Work out the finished part from the listing and answer in its coordinate system (mm). Face numbers are marked on the shaded views. Coordinates: 2 decimals unless noted, no trailing zeros. Write each loop counter-clockwise with the first axis right and the second up, starting at its lowest first coordinate (ties: lowest second). Pieces come first, ordered by that corner, then holes. Notation, with made-up numbers: (22, 47.5) - (75, 47.5) arc R32 ccw to (75, 74.5) - close; hole circle Ø2 at (41, 22). An arc over 180 degrees is marked (long way). Answer as a JSON object with one key per item and string values. Group by question number.
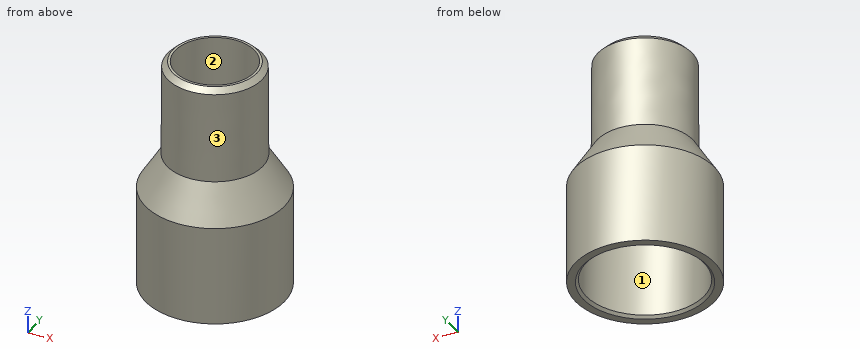
from build123d import *

# Parameters (mm, degrees)
F2_SIZE = 2
F3_SIZE = 1


with BuildPart() as f1:
    # F0 (on Front) → F1 (revolve)
    with BuildSketch(Plane.XZ):
        Polygon((22.5, 38), (22.5, 0), (26.5, 0), (26.5, 38), (18.2, 51.423181), (18, 88), (15.08, 88), (15.08, 50), align=None)
    revolve(axis=Axis((0, 0, 38.390822), (0, 0, 1)))

    # F2
    f2_edges = [f1.edges().sort_by_distance(p)[0] for p in [
        (-18, 0, 88),
    ]]
    chamfer(f2_edges, length=F2_SIZE)

    # F3
    f3_edges = [f1.edges().sort_by_distance(p)[0] for p in [
        (-22.5, 0, 0),
    ]]
    chamfer(f3_edges, length=F3_SIZE)


solid = f1.part
Q1. Section A-A on z = 33 is taken. Determine the outline of the cut face in (x, y).
Q2. For a pull along Y with two mould halves and no side action, classify the marked faces 1, 2 and 3 as +Y half, -Y half, draft (parallel to the pull), parting line (faces both ways), or undercut.
Q3. Section B-B on z = 66 is taken. Determine the outline of the cut face in (x, y), plus the area to 3 significant figures.
Q4. Flat-ended cylindrical pins translate along their axes: pin 1 Ø12 at (x, y) = (-8, -2) entering from -Z; pin 2 Ø2 at (y, z) = (-2.5, 59.5) entering from -X; pin 3 Ø5 at (x, y) = (11, -14) entering from -Z; pin 4 Ø3 at (x, z) = (16, 41) entering from +Y. Find the tip coordinate at first contact, or state that the pin passes through.
Q5. Consider L1, parallel to Y at x = 0, z = 17; L2, parallel to Y at x = 6, z = 70.5; L3, parallel to X at y = -4.5, z = 25.5. Determine where each line is inside the solid, lowest interval first. Write a range as from..to.
Numbers:
{
 "1": {"outline": "circle Ø53 at (0, 0); hole circle Ø45 at (0, 0)"},
 "2": {"face 1": "undercut", "face 2": "undercut", "face 3": "parting line"},
 "3": {"outline": "circle Ø36.24 at (0, 0); hole circle Ø30.16 at (0, 0)", "area": "317 mm²"},
 "4": {"pin 1": "passes through", "pin 2": "stops at x = -18.09", "pin 3": "stops at z = 41.55", "pin 4": "stops at y = 20.42"},
 "5": {"L1": "y = -26.5..-22.5, 22.5..26.5", "L2": "y = -17.07..-13.83, 13.83..17.07", "L3": "x = -26.12..-22.05, 22.05..26.12"}
}
